Work out the finished part from the listing and answer in its coordinate system (mm). A direction names the side the tool comes from. Round coordinates to 2 decimals unless told otherwise and drop trailing zeros. Loops run counter-clockwise (first coordinate to the right, second up) from the corner with the lowest first, then second, coordinate; pieces in that order, holes last. Notation, with made-up numbers: (69, 85.25) - (91, 85.25) arc R22 ccw to (91, 116.25) - close; hole circle Ø2 at (-35.75, 24). An arc over 180 degrees is marked (long way). Answer as CSV lines item,"result". Start each with the question number.
Q1. Section C-C on y = 3.45 is taken. Write down the section's boundary in (x, z).
Q2. Section A-A on z = 0 is taken. Write down the section's boundary in (x, y).
Q3. For faces 1 (the face through (-2.777, 4.479, 6.697)), 2 (the face through (1.802, 0.493, 5.723)), 3 (the face through (2.748, 1.74, 8.727)), determine the directions among +Z, -Z, +X, -X, +Y, -Y from which every point of the face is accessible in a straight line to the end or side of a thin tool.
Q4. Straight lines are drawn through the part: L1, parallel to Z at x = -0.25, y = 5.2; L2, parallel to Y at x = 0.5, z = -6.5. For each, find the intervals that lie inside material, in ascending order. Write a range as [from, to].
Q5. Each of these flat-tipped pins is pushed along its axis until it touches: pin 1 Ø1.5 at (x, z) = (-6.5, -5) entering from -Y; pin 2 Ø1 at (y, z) = (4, 1.5) entering from +X; pin 3 Ø2 at (x, y) = (4, 2.5) entering from +Z. Where does it stop, or does it pass through?
Q6. Section B-B on x = 0 is taken. Write down the section's boundary in (y, z).
```python
from build123d import *

# Parameters (mm, degrees)
SKETCH5_R           = 6
BOSS_EXTRUDE3_DEPTH = 1
SKETCH6_R           = 9.15
BOSS_EXTRUDE4_DEPTH = 2
CHAMFER1_SIZE       = 0.5
CHAMFER1_SIZE2      = 0.866025404
SKETCH7_R           = 7.25
BOSS_EXTRUDE5_DEPTH = 3


with BuildPart() as part:
    # Sketch5 → Boss-Extrude3 (new body)
    with BuildSketch(Plane(origin=(0, 0, 0), x_dir=(1, 0, 0), z_dir=(0, 1, 0))):
        with Locations(Location((0, 0, 0), (0, 0, 270))):
            Circle(SKETCH5_R)
    extrude(amount=BOSS_EXTRUDE3_DEPTH)

    # Sketch6 → Boss-Extrude4 (add)
    with BuildSketch(Plane(origin=(0, 1, 0), x_dir=(1, 0, 0), z_dir=(0, 1, 0))):
        with Locations(Location((0, 0, 0), (0, 0, 270))):
            Circle(SKETCH6_R)
    extrude(amount=BOSS_EXTRUDE4_DEPTH)

    # Chamfer1
    chamfer1_edges = [part.edges().sort_by_distance(p)[0] for p in [
        (0, 3, -9.15),
    ]]
    chamfer1_side = [part.faces().sort_by_distance(p)[0] for p in [
        (0, 2, -9.15),
    ]]
    chamfer(chamfer1_edges, length=CHAMFER1_SIZE, length2=CHAMFER1_SIZE2, reference=chamfer1_side[0])

    # Sketch7 → Boss-Extrude5 (add)
    with BuildSketch(Plane(origin=(0, 3, 0), x_dir=(1, 0, 0), z_dir=(0, 1, 0))):
        with Locations(Location((0, 0, 0), (0, 0, 270))):
            Circle(SKETCH7_R)
    extrude(amount=BOSS_EXTRUDE5_DEPTH)


solid = part.part
```
Findings:
1,outline,"circle Ø14.5 at (0, 0)"
2,outline,"(-9.15, 1) - (-6, 1) - (-6, 0) - (6, 0) - (6, 1) - (9.15, 1) - (9.15, 2.5) - (8.28, 3) - (7.25, 3) - (7.25, 6) - (-7.25, 6) - (-7.25, 3) - (-8.28, 3) - (-9.15, 2.5) - close"
3,face 1,"+Y"
3,face 2,"-Y"
3,face 3,"+Y, -Y"
4,L1,"z = [-7.25, 7.25]"
4,L2,"y = [1, 6]"
5,pin 1,"stops at y = 1"
5,pin 2,"stops at x = 7.18"
5,pin 3,"stops at z = 8.64"
6,outline,"(0, -6) - (1, -6) - (1, -9.15) - (2.5, -9.15) - (3, -8.28) - (3, -7.25) - (6, -7.25) - (6, 7.25) - (3, 7.25) - (3, 8.28) - (2.5, 9.15) - (1, 9.15) - (1, 6) - (0, 6) - close"
